Design review of the part shown in the three views and the two pictorial views. Dimensions are in mm from the part's minimum x, y and z. A direction names the side the tool comes from. Give positions to 0.01 mm unless a question says otherwise; leave off trailing zeros. Order: outer loops, then holes, each group sorted by start corner. A loop starts at its lowest first (then second) coordinate and runs counter-clockwise, first axis right, second up. Notation, with made-up numbers: (71, -29.5) - (79, -29.5) arc R32 ccw to (79, 0.5) - close; hole circle Ø4 at (-40, -35). An arc over 180 degrees is marked (long way). Put each result on its own line as item: value.
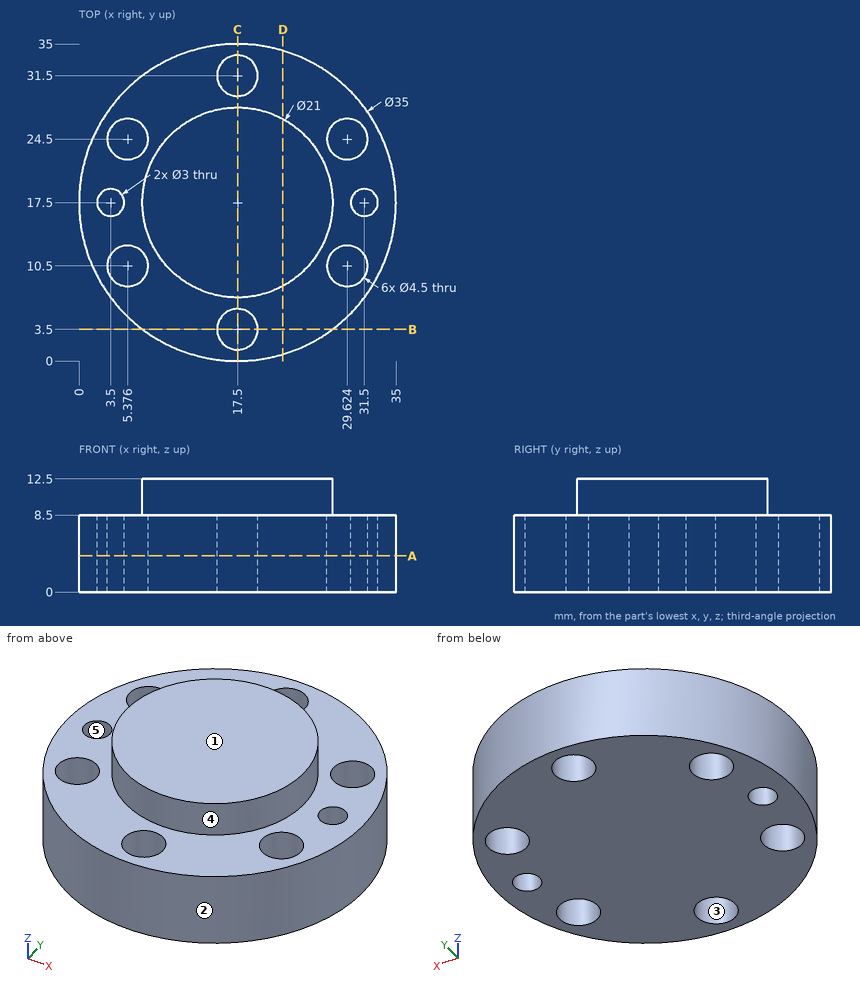
(1) Take a section at B-B, the plane y = 3.5. Write out the cut boundary in (x, z), then the cut area to 3 significant figures.
The answers:
outline: (7, 0) - (15.25, 0) - (15.25, 8.5) - (7, 8.5) - close; (19.75, 0) - (28, 0) - (28, 8.5) - (19.75, 8.5) - close
area: 140 mm^2
(2) Take a section at D-D, the plane x = 22.5. Write out the cut boundary in (y, z), then the cut area to 3 significant figures.
The answers:
outline: (0.73, 0) - (34.27, 0) - (34.27, 8.5) - (26.73, 8.5) - (26.73, 12.5) - (8.27, 12.5) - (8.27, 8.5) - (0.73, 8.5) - close
area: 359 mm^2
(3) The part is to be moulded in two halves that separate along Y. For the marked faces 1, 2 and 3, say which applies: pulls with the +Y half, pulls with the -Y half, needs draft (parallel to the pull), parting line crosses it, or undercut.
The answers:
face 1: needs draft
face 2: parting line crosses it
face 3: undercut
(4) Clearance check with flat-ended pins moving along their axes: pin 1 Ø5 at (y, z) = (24.5, 8) entering from +X; pin 2 Ø5 at (x, y) = (5.38, 10.5) entering from -Z; pin 3 Ø2 at (x, z) = (28.5, 7) entering from +Y; pin 4 Ø3 at (y, z) = (7.5, 4.5) entering from -X. State where each tip first meets the part, or that it passes through.
The answers:
pin 1: x = 34.41
pin 2: z = 0
pin 3: y = 31.86
pin 4: x = 2.2
(5) Take a section at C-C, the plane x = 17.5. Write out the cut boundary in (y, z).
The answers:
outline: (0, 0) - (1.25, 0) - (1.25, 8.5) - (0, 8.5) - close; (5.75, 0) - (29.25, 0) - (29.25, 8.5) - (28, 8.5) - (28, 12.5) - (7, 12.5) - (7, 8.5) - (5.75, 8.5) - close; (33.75, 0) - (35, 0) - (35, 8.5) - (33.75, 8.5) - close
(6) Wall thickness on L1, parallel to Y at x = 17.5, z = 5.75; L2, parallel to Y at x = 3.5, z = 3.5 (1 decimal); L3, parallel to Y at x = 6, z = 7.5: over which ranges is each line inside the solid? List them lowest first.
The answers:
L1: 0 to 1.25, 5.75 to 29.25, 33.75 to 35
L2: 7 to 9.3, 11.7 to 16, 19 to 23.3, 25.7 to 28
L3: 4.31 to 8.34, 12.66 to 22.34, 26.66 to 30.69
(7) For the marked faces 4 and 5, list the 3-axis set-ups (+Z, -Z, +X, -X, +Y, -Y) from which the entire face can be reached by the end or side of a thin tool; tool diameter is ignored.
The answers:
face 4: +Z
face 5: +Z, -Z
(8) Take a section at A-A, the plane z = 4. Count the separate pieces of the cut face and the enclosed holes in it.
The answers:
separate pieces: 1
enclosed holes: 8
